from build123d import *
from OCP.BRepFilletAPI import BRepFilletAPI_MakeChamfer

# Parameters (mm, degrees)
BOSS_EXTRUDE1_DEPTH      = 6
SKETCH2_W                = 15.427107808
SKETCH2_H                = 31.27334873
BOSS_EXTRUDE2_DEPTH      = 8
CUT_EXTRUDE1_DEPTH       = 23.360780376
CUT_EXTRUDE2_DEPTH       = 5
CHAMFER1_SIZE            = 1
CHAMFER1_SIZE2           = 0.577350269
CUT_EXTRUDE4_DEPTH       = 20.183443357
SKETCH17_W               = 2
SKETCH17_H               = 3.5
BOSS_EXTRUDE3_DEPTH      = 8
CIRPATTERN1_COUNT        = 2
FILLET3_R                = 2
SKETCH20_W               = 13.713553904
SKETCH20_H               = 1.226825257
CUT_EXTRUDE5_DEPTH       = 23.90339353
F_4_0_4_DIAMETER_HOLE3_D = 4
M3X0_5_TAPPED_HOLE1_D    = 2.5
F_4_0_4_DIAMETER_HOLE5_D = 4


with BuildPart() as part:
    # Sketch1 → Boss-Extrude1 (new body)
    with BuildSketch(Plane.XY):
        with BuildLine():
            Line((2.001816135, 13.723643263), (-7.525291673, -11.649705468))
            ThreePointArc((-7.525291673, -11.649705468), (-5.800522802, -15.448412135), (-2.001816135, -13.723643263))
            Line((-2.001816135, -13.723643263), (7.525291673, 11.649705468))
            ThreePointArc((7.525291673, 11.649705468), (5.800522802, 15.448412135), (2.001816135, 13.723643263))
        make_face()
    extrude(amount=BOSS_EXTRUDE1_DEPTH)

    # Sketch2 → Boss-Extrude2 (add)
    with BuildSketch(Plane(origin=(0, 0, 0), x_dir=(-1, 0, 0), z_dir=(0, 0, -1))):
        Rectangle(SKETCH2_W, SKETCH2_H)
    extrude(amount=BOSS_EXTRUDE2_DEPTH)

    # Sketch3 → Cut-Extrude1 (cut, through all)
    with BuildSketch(Plane.XY.offset(6)):
        with BuildLine():
            Line((1.943905795, 9.444408677), (-4.752452679, -8.389864035))
            ThreePointArc((-4.752452679, -8.389864035), (-3.875451558, -10.321409798), (-1.943905795, -9.444408677))
            Line((-1.943905795, -9.444408677), (4.752452679, 8.389864035))
            ThreePointArc((4.752452679, 8.389864035), (3.875451558, 10.321409798), (1.943905795, 9.444408677))
        make_face()
    extrude(amount=-CUT_EXTRUDE1_DEPTH, mode=Mode.SUBTRACT)

    # Sketch4 → Cut-Extrude2 (cut)
    with BuildSketch(Plane.XY.offset(6)):
        with BuildLine():
            Line((2.001816135, 13.723643263), (-7.525291673, -11.649705468))
            ThreePointArc((-7.525291673, -11.649705468), (-5.800522802, -15.448412135), (-2.001816135, -13.723643263))
            Line((-2.001816135, -13.723643263), (7.525291673, 11.649705468))
            ThreePointArc((7.525291673, 11.649705468), (5.800522802, 15.448412135), (2.001816135, 13.723643263))
        make_face()
        with BuildLine():
            Line((2.189052594, 13.653340287), (-7.338055214, -11.720008444))
            ThreePointArc((-7.338055214, -11.720008444), (-5.730219825, -15.261175676), (-2.189052594, -13.653340287))
            Line((-2.189052594, -13.653340287), (7.338055214, 11.720008444))
            ThreePointArc((7.338055214, 11.720008444), (5.730219825, 15.261175676), (2.189052594, 13.653340287))
        make_face(mode=Mode.SUBTRACT)
    extrude(amount=-CUT_EXTRUDE2_DEPTH, mode=Mode.SUBTRACT)

    # Chamfer1: one chamfer whose edges measure the first distance from different faces: ONE call of the kernel's chamfer builder (chamfer() names one face for all edges)
    chamfer1_edges_1 = [part.edges().sort_by_distance(p)[0] for p in [
        (2.57450131, -0.966665922, 6),
    ]]
    chamfer1_side_1 = [part.faces().sort_by_distance(p)[0] for p in [
        (2.57450131, -0.966665922, 3.5),
    ]]
    chamfer1_edges_2 = [part.edges().sort_by_distance(p)[0] for p in [
        (5.730219825, 15.261175676, 6),
    ]]
    chamfer1_side_2 = [part.faces().sort_by_distance(p)[0] for p in [
        (5.730219825, 15.261175676, 3.5),
    ]]
    chamfer1_edges_3 = [part.edges().sort_by_distance(p)[0] for p in [
        (-2.57450131, 0.966665922, 6),
    ]]
    chamfer1_side_3 = [part.faces().sort_by_distance(p)[0] for p in [
        (-2.57450131, 0.966665922, 3.5),
    ]]
    chamfer1_edges_4 = [part.edges().sort_by_distance(p)[0] for p in [
        (-5.730219825, -15.261175676, 6),
    ]]
    chamfer1_side_4 = [part.faces().sort_by_distance(p)[0] for p in [
        (-5.730219825, -15.261175676, 3.5),
    ]]
    chamfer1 = BRepFilletAPI_MakeChamfer(part.part.solid().wrapped)
    for e in chamfer1_edges_1:
        chamfer1.Add(CHAMFER1_SIZE, CHAMFER1_SIZE2, e.wrapped, chamfer1_side_1[0].wrapped)  # the first distance lies on this face
    for e in chamfer1_edges_2:
        chamfer1.Add(CHAMFER1_SIZE, CHAMFER1_SIZE2, e.wrapped, chamfer1_side_2[0].wrapped)  # the first distance lies on this face
    for e in chamfer1_edges_3:
        chamfer1.Add(CHAMFER1_SIZE, CHAMFER1_SIZE2, e.wrapped, chamfer1_side_3[0].wrapped)  # the first distance lies on this face
    for e in chamfer1_edges_4:
        chamfer1.Add(CHAMFER1_SIZE, CHAMFER1_SIZE2, e.wrapped, chamfer1_side_4[0].wrapped)  # the first distance lies on this face
    add(Compound.cast(chamfer1.Shape()), mode=Mode.REPLACE)

    # Sketch11 → Cut-Extrude4 (cut, through all)
    with BuildSketch(Plane.XY):
        with BuildLine():
            Line((4.763553904, 15.636674365), (7.713553904, 15.636674365))
            Line((7.713553904, 15.636674365), (7.713553904, 12.686674365))
            ThreePointArc((7.713553904, 12.686674365), (6.849518908, 14.77263937), (4.763553904, 15.636674365))
        make_face()
        with BuildLine():
            Line((-7.713553904, -12.686674365), (-7.713553904, -15.636674365))
            Line((-7.713553904, -15.636674365), (-4.763553904, -15.636674365))
            ThreePointArc((-4.763553904, -15.636674365), (-6.849518908, -14.77263937), (-7.713553904, -12.686674365))
        make_face()
    extrude(amount=-CUT_EXTRUDE4_DEPTH, mode=Mode.SUBTRACT)

    # Sketch17 → Boss-Extrude3 (add, through all)
    with BuildSketch(Plane.XY):
        with BuildLine():
            Line((7.713553904, 12.686674365), (7.713553904, -15.636674365))
            Line((7.713553904, -15.636674365), (9.713553904, -15.636674365))
            Line((9.713553904, -15.636674365), (9.713553904, 13.979159118))
            Line((9.713553904, 13.979159118), (5.800522802, 15.448412135))
            ThreePointArc((5.800522802, 15.448412135), (7.188585682, 14.366472233), (7.713553904, 12.686674365))
        make_face()
        with BuildLine():
            ThreePointArc((4.763553904, 15.636674365), (5.290513855, 15.589227243), (5.800522802, 15.448412135))
            Line((5.800522802, 15.448412135), (4, 16.12446696))
            Line((4, 16.12446696), (4, 19.136674365))
            Line((4, 19.136674365), (-7.713553904, 19.136674365))
            Line((-7.713553904, 19.136674365), (-7.713553904, 15.636674365))
            Line((-7.713553904, 15.636674365), (4.763553904, 15.636674365))
        make_face()
        with Locations((-8.713553904, 17.386674365)):
            Rectangle(SKETCH17_W, SKETCH17_H)
    boss_extrude3 = extrude(amount=-BOSS_EXTRUDE3_DEPTH)

    # CirPattern1: Boss-Extrude3 ×2 about axis
    cirpattern1_axis = Axis((0, 0, 0), (0, 0, 1))
    for i in range(1, CIRPATTERN1_COUNT):
        add(boss_extrude3.rotate(cirpattern1_axis, i * 360 / CIRPATTERN1_COUNT))

    # Fillet3
    fillet3_edges = [part.edges().sort_by_distance(p)[0] for p in [
        (4, 16.12446696, -4),
        (-4, -16.12446696, -4),
    ]]
    fillet(fillet3_edges, radius=FILLET3_R)

    # Sketch20 → Cut-Extrude5 (cut, through all)
    with BuildSketch(Plane.XY):
        with Locations((2.856776952, -18.523261737)):
            Rectangle(SKETCH20_W, SKETCH20_H)
    extrude(amount=-CUT_EXTRUDE5_DEPTH, mode=Mode.SUBTRACT)

    # 4.0 _4_ Diameter Hole3 (through all)
    with Locations(Plane(origin=(-9.713553904, 2.428457005, -0.24781288), x_dir=(0, 0, 1), z_dir=(-1, 0, 0))):
        with Locations((-3.75218712, 3.921542995), (-3.75218712, -8.778457005), (-3.75218712, -2.428457005)):
            Hole(F_4_0_4_DIAMETER_HOLE3_D / 2)

    # M3x0.5 Tapped Hole1 (through all)
    with Locations(Plane.XY.offset(6)):
        with Locations((-4.768557373, -12.7), (4.768557373, 12.7)):
            Hole(M3X0_5_TAPPED_HOLE1_D / 2)

    # 4.0 _4_ Diameter Hole5 (through all)
    with Locations(Plane.XY):
        with Locations((-4.768557373, 12.7), (4.768557373, -12.7)):
            Hole(F_4_0_4_DIAMETER_HOLE5_D / 2)


solid = part.part
Could you check a few things on this model? Use its own coordinates, in mm. A direction names the side the tool comes from. Round coordinates to 2 decimals unless told otherwise and drop trailing zeros. Order: outer loops, then holes, each group sorted by start corner. A loop starts at its lowest first (then second) coordinate and runs counter-clockwise, first axis right, second up.
(1) Imagine slicing it at D-D (y = 9). Write out the boundary of the cut face in (x, z), plus the area to 3 significant figures.
Response values:
outline: (-9.71, -8) - (1.78, -8) - (1.78, 6) - (1.06, 6) - (0.44, 5) - (0.44, 1) - (0.23, 1) - (0.23, 0) - (-9.71, 0) - close; (4.85, -8) - (9.71, -8) - (9.71, 0) - (6.53, 0) - (6.53, 1) - (6.32, 1) - (6.32, 5) - (5.7, 6) - (4.85, 6) - close
area: 148 mm2
(2) Imagine slicing it at B-B (y = 0.5). Write out the boundary of the cut face in (x, z).
Response values:
outline: (-9.71, -8) - (-1.41, -8) - (-1.41, -5.94) - (-9.71, -5.94) - close; (-9.71, -2.06) - (-1.41, -2.06) - (-1.41, 6) - (-2.13, 6) - (-2.75, 5) - (-2.75, 1) - (-2.96, 1) - (-2.96, 0) - (-9.71, 0) - close; (1.79, -8) - (9.71, -8) - (9.71, -5.94) - (1.79, -5.94) - close; (1.79, -2.06) - (9.71, -2.06) - (9.71, 0) - (3.34, 0) - (3.34, 1) - (3.13, 1) - (3.13, 5) - (2.51, 6) - (1.79, 6) - close
(3) Which directions (+Z, -Z, +X, -X, +Y, -Y) give clear straight access to the entire face, cutting with the end or side of a thin tool? Please do faces 1 (the flat face through (4, 18, -4)), 2 (the flat face through (1.36, -0.65, -0.9)), 3 (the cylindrical face through (-4.35, -16.38, -4.06)), 4 (the flat face through (-2.51, 1.14, 3.03)), 5 (the flat face through (2.51, -1.14, 3.03)).
Response values:
face 1: +Z, -Z, +X, +Y
face 2: +Z, -Z
face 3: +Z, -Z, -X, -Y
face 4: +Z, -X, +Y
face 5: +Z, +X, -Y
(4) Imagine slicing it at A-A (z = 4.25). Write out the boundary of the cut face in (x, y).
Response values:
outline: (-7.34, -11.72) arc R2.75 ccw to (-2.19, -13.65) - (7.34, 11.72) arc R2.75 ccw to (2.19, 13.65) - close; hole circle Ø2.5 at (-4.77, -12.7); hole (-4.75, -8.39) arc R1.5 ccw to (-1.94, -9.44) - (4.75, 8.39) arc R1.5 ccw to (1.94, 9.44) - close; hole circle Ø2.5 at (4.77, 12.7)
(5) I'm going to push flat-ended pins straight in: pin 1 (6 mm diameter, centred on x = -0.5, z = 2, fed in from -Y); pin 2 (2 mm diameter, centred on x = 5.5, y = -6.5, fed in from +Z); pin 3 (1.5 mm diameter, centred on x = -3.5, y = 0, fed in from +Z); pin 4 (1.8 mm diameter, centred on y = 18, z = -5, fed in from +X). Where does each tip first touch, or does it pass through?
Response values:
pin 1: stops at y = -17.91
pin 2: stops at z = 0
pin 3: stops at z = 5.39
pin 4: stops at x = 4.04
(6) If we mould it in two halves opening along Y, with no side actions, what happens to faces 6 (the cylindrical face through (-3.91, -10.31, -0.9)), 7 (the flat face through (2.7, -1.2, 0.5)), 8 (the flat face through (6, -5, 0)), 9 (the cylindrical face through (-7.121, -4.367, -3.74))? For each: released by +Y, released by -Y, zero draft, split by the parting line, or undercut.
Response values:
face 6: undercut
face 7: released by -Y
face 8: zero draft
face 9: undercut
(7) Please list where these lines run through material, in increasing order: line 1 along Z through (x, y) = (6.5, 6.35); line 2 along Y through (x, z) = (5, -3); line 3 along X through (y, z) = (13, -3).
Response values:
line 1: z = -8 to -6, -2 to 0
line 2: y = -17.91 to -14.69, -10.71 to -8.08, -4.62 to -1.73, 1.73 to 4.62, 8.08 to 11.47, 13.93 to 15.78
line 3: x = -9.71 to -6.75, -2.79 to 3.56, 5.98 to 9.71
(8) Imagine slicing it at C-C (z = -7). Write out the boundary of the cut face in (x, y).
Response values:
outline: (-9.71, -13.98) - (-5.3, -15.64) arc R2 cw to (-4, -17.51) - (-4, -17.91) - (9.71, -17.91) - (9.71, 13.98) - (5.3, 15.64) arc R2 cw to (4, 17.51) - (4, 19.14) - (-9.71, 19.14) - close; hole circle Ø4 at (-4.77, 12.7); hole circle Ø2.5 at (-4.77, -12.7); hole (-4.75, -8.39) arc R1.5 ccw to (-1.94, -9.44) - (4.75, 8.39) arc R1.5 ccw to (1.94, 9.44) - close; hole circle Ø4 at (4.77, -12.7); hole circle Ø2.5 at (4.77, 12.7)
